Model file for the job. Use its own axes, mm. A direction names the side the tool comes from. Round coordinates to 2 decimals unless told otherwise and drop trailing zeros. Order: outer loops, then holes, each group sorted by start corner. A loop starts at its lowest first (then second) coordinate and runs counter-clockwise, first axis right, second up. Notation, with made-up numbers: (-9, -11) - (34, -11) arc R12 cw to (34, -1) - close; hole circle Ø9 at (18, 71.5). An arc over 180 degrees is marked (long way). Write item = value, one per line. Start each with the question number.
from build123d import *

# Parameters (mm, degrees)
CROQUIS2_W            = 5
CROQUIS2_H            = 5
CORTAR_EXTRUIR1_DEPTH = 24.290725622


with BuildPart() as part:
    # Croquis1 → Revolución1 (revolve)
    with BuildSketch(Plane(origin=(0, 0, 0), x_dir=(0, 0, -1), z_dir=(1, 0, 0)), mode=Mode.PRIVATE) as revoluci_n1_sk:
        with BuildLine():
            Line((0, 8.5), (0, 10.05))
            Line((0, 10.05), (0.2, 10.25))
            Line((0.2, 10.25), (5.8, 10.25))
            Line((5.8, 10.25), (6, 10.05))
            Line((6, 10.05), (6, 9.565))
            ThreePointArc((6, 9.565), (6.439339828, 8.504339828), (7.5, 8.065))
            Line((7.5, 8.065), (18.03, 8.065))
            Line((18.03, 8.065), (18.23, 7.865))
            Line((18.23, 7.865), (18.23, 6.2))
            Line((18.23, 6.2), (18.03, 6))
            Line((18.03, 6), (2.5, 6))
            Line((2.5, 6), (0, 8.5))
        make_face()
    revolve(revoluci_n1_sk.sketch.rotate(Axis((0, 0, 0), (0, 0, -1)), 90), axis=Axis((0, 0, 0), (0, 0, -1)))

    # Croquis2 → Cortar-Extruir1 (cut, through all)
    with BuildSketch(Plane(origin=(0, 0, 0), x_dir=(1, 0, 0), z_dir=(0, 1, 0))):
        with Locations((0, 15.73)):
            Rectangle(CROQUIS2_W, CROQUIS2_H)
    extrude(amount=-CORTAR_EXTRUIR1_DEPTH, mode=Mode.SUBTRACT)


solid = part.part
Item 1: Saw through at A-A, the plane x = 0. Give the cut face in (y, z) (3 decimals), then the cut area to 3 significant figures.
Item 2: Probe L1, parallel to Y at x = 0, z = -10.75 (3 decimals); L2, parallel to X at y = -0.25, z = -12.5; L3, parallel to Y at x = 0, z = -5.25. List the from-to ranges inside material, lowest first.
Item 3: Mould opens along X. For faces 1 (the face through (5.69, 2.36, -2.34)), 2 (the face through (7.5, -4.5, 0)), 3 (the face through (-1.748, 7.873, -12.839)) say: +X half, -X half, draft (parallel to the pull), parting line (faces both ways), or undercut.
Item 4: Saw through at D-D, the plane z = -16.5. Give the cut face in (x, y) (3 decimals), then the cut area to 3 significant figures.
Item 5: Saw through at B-B, the plane y = 0. Give the cut face in (x, z) (3 decimals), then the cut area to 3 significant figures.
Item 6: Drop flat-ended pins along their axis: pin 1 (1.5 mm diameter, centred on x = 7.5, z = -16, fed in from +Y); pin 2 (6 mm diameter, centred on y = 8, z = -6, fed in from +X); pin 3 (7 mm diameter, centred on x = 0, y = 0, fed in from -Z); pin 4 (8 mm diameter, centred on y = -3, z = -12, fed in from -X) (3 decimals). Give the stop position or say it passes through.
Item 7: Saw through at C-C, the plane z = -9.5. Give the cut face in (x, y) (3 decimals), then the cut area to 3 significant figures.
Item 8: Which spindle directions (+Z, -Z, +X, -X, +Y, -Y) get a long thin tool onto all of the face, cutting with end or side? Do faces 4 (the face through (9, 4, -6)), 5 (the face through (2.769, 5.323, -10.156)), 6 (the face through (0, -7, -13.23)). Say none if no direction does.
Check sheet entries:
q1.outline = (-10.25, -5.8) - (-10.05, -6) - (-9.565, -6) arc R1.5 cw to (-8.065, -7.5) - (-8.065, -13.23) - (-6, -13.23) - (-6, -2.5) - (-8.5, 0) - (-10.05, 0) - (-10.25, -0.2) - close; (6, -18.03) - (6.2, -18.23) - (7.865, -18.23) - (8.065, -18.03) - (8.065, -7.5) arc R1.5 cw to (9.565, -6) - (10.05, -6) - (10.25, -5.8) - (10.25, -0.2) - (10.05, 0) - (8.5, 0) - (6, -2.5) - close
q1.area = 85.8 mm2
q2.L1 = -8.065 to -6, 6 to 8.065
q2.L2 = -8.06 to -5.99, 5.99 to 8.06
q2.L3 = -10.25 to -6, 6 to 10.25
q3.face_1 = undercut
q3.face_2 = draft
q3.face_3 = parting line
q4.outline = (-2.5, -7.668) - (-2.5, -5.454) arc R6 cw (long way) to (2.5, -5.454) - (2.5, -7.668) arc R8.065 ccw (long way) to start
q4.area = 80.7 mm2
q5.outline = (-10.25, -5.8) - (-10.05, -6) - (-9.565, -6) arc R1.5 cw to (-8.065, -7.5) - (-8.065, -18.03) - (-7.865, -18.23) - (-6.2, -18.23) - (-6, -18.03) - (-6, -2.5) - (-8.5, 0) - (-10.05, 0) - (-10.25, -0.2) - close; (6, -18.03) - (6.2, -18.23) - (7.865, -18.23) - (8.065, -18.03) - (8.065, -7.5) arc R1.5 cw to (9.565, -6) - (10.05, -6) - (10.25, -5.8) - (10.25, -0.2) - (10.05, 0) - (8.5, 0) - (6, -2.5) - close
q5.area = 96.1 mm2
q6.pin_1 = 4.41
q6.pin_2 = 8.94
q6.pin_3 = through
q6.pin_4 = -8.065
q7.outline = circle Ø16.13 at (0, 0); hole circle Ø12 at (0, 0)
q7.area = 91.2 mm2
q8.face_4 = -Z
q8.face_5 = +Z, -Z
q8.face_6 = -Z, -Y
